For this review, use the dimensioned drawing (mm, ordinates from the lowest corner) and the shaded views. A direction names the side the tool comes from. Round coordinates to 2 decimals unless told otherwise and drop trailing zeros. Loops run counter-clockwise (first coordinate to the right, second up) from the corner with the lowest first, then second, coordinate; pieces in that order, holes last. Notation, with made-up numbers: (-35, 89.25) - (-4, 89.25) arc R20 cw to (-4, 114.25) - close; hole circle Ø7 at (73.5, 52.25). An arc over 180 degrees is marked (long way). Answer as CSV lines item,"result". Start each with the question number.
(1) Consider section D-D (z = 27). Give the boundary of the cut face in (x, y) (1 decimal).
(2) Consider section A-A (z = 34). Give the boundary of the cut face in (x, y) (1 decimal).
(3) Consider section C-C (x = 21). Give the boundary of the cut face in (y, z), and give its area (3 significant figures).
(4) Wall thickness on L1, parallel to Y at x = 43.5, z = 42.5; L2, parallel to Y at x = 27, z = 36; L3, parallel to Z at x = 30, y = 40: over which ranges is each line inside the solid? List them lowest first.
(5) Consider section B-B (y = 44). Give the boundary of the cut face in (x, z).
(6) For the marked faces 5, 6 and 7, list the 3-axis set-ups (+Z, -Z, +X, -X, +Y, -Y) from which the entire face can be reached by the end or side of a thin tool; tool diameter is ignored.
(7) For P1, Ø10, axis at x = 53.5, z = 10.5, coming from the -Y side; P2, Ø14, axis at x = 29.5, y = 35.5, coming from the +Z side; P3, Ø1.5, axis at y = 56, z = 28, coming from the +X side, all flat-tipped, find the tip position at first contact; note any pin that passes through.
(8) Mouldability with a two-part tool opening along X and no side actions: class the marked faces 1, 2, 3 and 4 as released by +X, released by -X, zero draft, split by the parting line, or undercut.
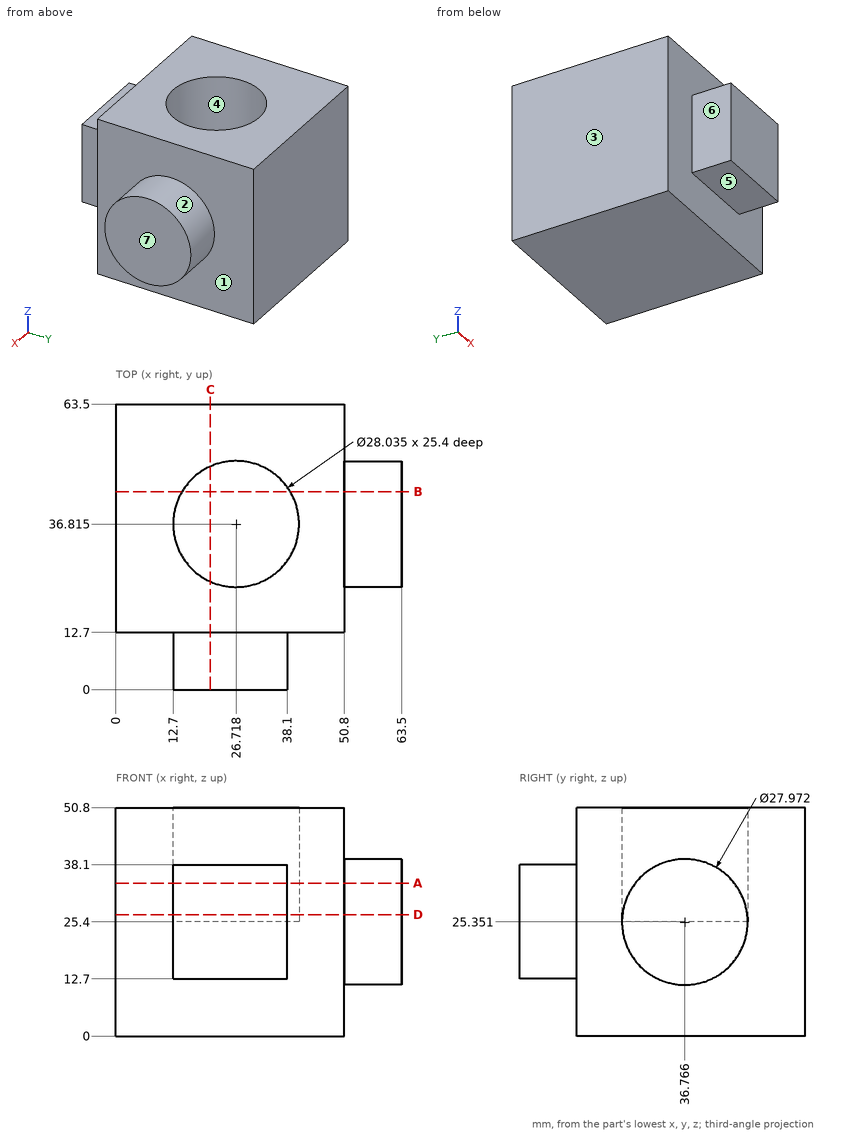
Determined:
1,outline,"(0, 12.7) - (12.7, 12.7) - (12.7, 0) - (38.1, 0) - (38.1, 12.7) - (50.8, 12.7) - (50.8, 22.9) - (63.5, 22.9) - (63.5, 50.7) - (50.8, 50.7) - (50.8, 63.5) - (0, 63.5) - close; hole circle Ø28 at (26.7, 36.8)"
2,outline,"(0, 12.7) - (12.7, 12.7) - (12.7, 0) - (38.1, 0) - (38.1, 12.7) - (50.8, 12.7) - (50.8, 25.8) - (63.5, 25.8) - (63.5, 47.8) - (50.8, 47.8) - (50.8, 63.5) - (0, 63.5) - close; hole circle Ø28 at (26.7, 36.8)"
3,outline,"(0, 12.7) - (12.7, 12.7) - (12.7, 0) - (63.5, 0) - (63.5, 50.8) - (49.61, 50.8) - (49.61, 25.4) - (24.02, 25.4) - (24.02, 50.8) - (12.7, 50.8) - (12.7, 38.1) - (0, 38.1) - close"
3,area,"2,250 mm^2"
4,L1,"y = 12.7 to 63.5"
4,L2,"y = 0 to 22.8, 50.83 to 63.5"
4,L3,"z = 0 to 25.4"
5,outline,"(0, 0) - (50.8, 0) - (50.8, 13.38) - (63.5, 13.38) - (63.5, 37.32) - (50.8, 37.32) - (50.8, 50.8) - (38.75, 50.8) - (38.75, 25.4) - (14.68, 25.4) - (14.68, 50.8) - (0, 50.8) - close"
6,face 5,"-Z, +X, -X, -Y"
6,face 6,"+Z, -Z, -X, -Y"
6,face 7,"+Z, -Z, +X, +Y, -Y"
7,P1,"stops at y = 12.7"
7,P2,"stops at z = 25.4"
7,P3,"stops at x = 50.8"
8,face 1,"released by +X"
8,face 2,"zero draft"
8,face 3,"released by -X"
8,face 4,"undercut"
